Part print with two shaded views. Sizes in mm from the minimum x, y, z corner. A direction names the side the tool comes from. Round coordinates to 2 decimals unless told otherwise and drop trailing zeros. Write each loop counter-clockwise with the first axis right and the second up, starting at its lowest first coordinate (ties: lowest second). Pieces come first, ordered by that corner, then holes. Notation, with made-up numbers: M -26,-18.75 L 8,-18.75 A20 cw 8,11.25 Z; hole C 0.25,63 d10. An arc over 180 degrees is marked long. Use one line per item in the form item = value. Start each with the question number.
Item 1: Mould opens along X. For the marked faces 1 and 2 say: +X half, -X half, draft (parallel to the pull), parting line (faces both ways), or undercut.
Item 2: Which spindle directions (+Z, -Z, +X, -X, +Y, -Y) get a long thin tool onto all of the face, cutting with end or side? Do the marked faces 3, 4 and 5. Say none if no direction does.
Item 3: Cut at A-A, the plane x = 16.8. Give the cut face in (y, z).
Item 4: Cut at C-C, the plane z = 3. Give the cut face in (x, y).
Item 5: Cut at D-D, the plane x = 2. Give the cut face in (y, z), then the cut area to 3 significant figures.
Item 6: Probe L1, parallel to X at y = 0.6, z = 5; L2, parallel to Y at x = 29.5, z = 2.75; L3, parallel to X at y = 3.75, z = 6.75. List the from-to ranges inside material, lowest first.
Item 7: Flat gauge pins, fed straight in: pin 1 Ø6 at (x, z) = (8, 3.5) entering from -Y; pin 2 Ø4 at (x, y) = (5, 4) entering from -Z; pin 3 Ø4 at (y, z) = (4, 5) entering from +X; pin 4 Ø5 at (x, z) = (20, 7) entering from +Y. Where does each tip first touch, or does it go through?
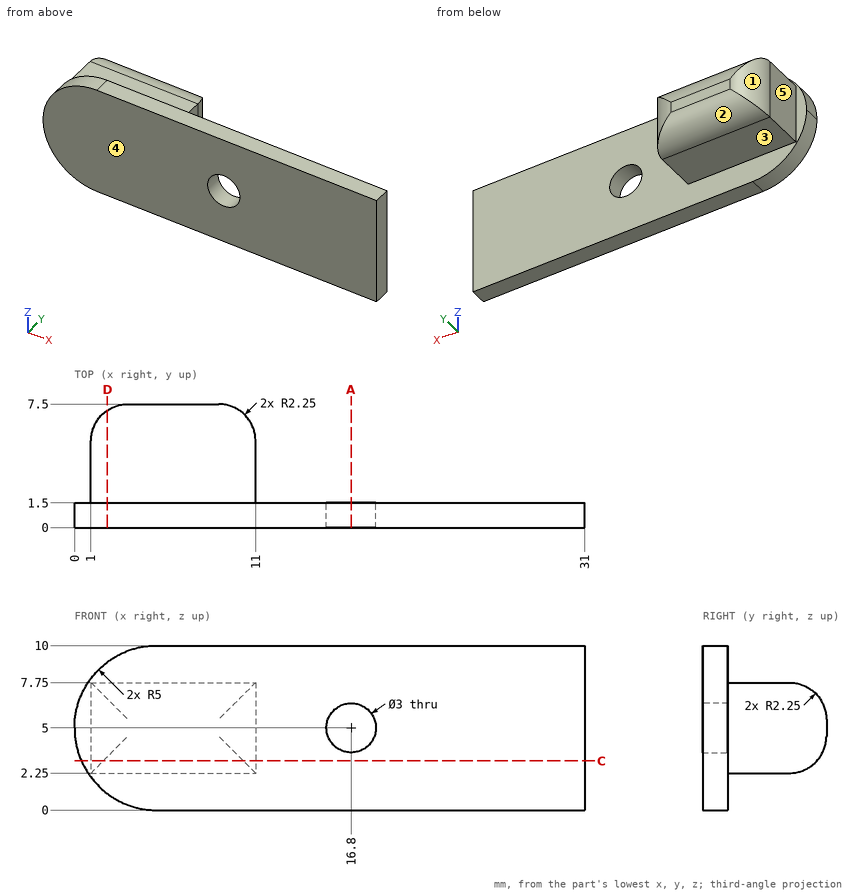
Model answer:
q1.face_1 = -X half
q1.face_2 = draft
q2.face_3 = -Z, +X, -X, +Y
q2.face_4 = +Z, -Z, +X, -X, -Y
q2.face_5 = +Z, -Z, -X, +Y
q3.outline = M 0,0 L 1.5,0 L 1.5,3.5 L 0,3.5 Z; M 0,6.5 L 1.5,6.5 L 1.5,10 L 0,10 Z
q4.outline = M 0.42,0 L 31,0 L 31,1.5 L 11,1.5 L 11,5.25 A2.25 ccw 10.25,6.93 L 1.75,6.93 A2.25 ccw 1,5.25 L 1,1.5 L 0.42,1.5 Z
q5.outline = M 0,1 L 1.5,1 L 1.5,2.25 L 5.25,2.25 A2.25 ccw 7.12,3.25 L 7.12,6.75 A2.25 ccw 5.25,7.75 L 1.5,7.75 L 1.5,9 L 0,9 Z
q5.area = 41.8 mm²
q6.L1 = 0 to 15.3, 18.3 to 31
q6.L2 = 0 to 1.5
q6.L3 = 1 to 11
q7.pin_1 = 0
q7.pin_2 = 2.25
q7.pin_3 = 11
q7.pin_4 = 1.5
